Design review of the part built by this model. Coordinates are the model's own, in mm. Face numbers are marked on the shaded views. A direction names the side the tool comes from. Give positions to 0.01 mm unless a question says otherwise; leave off trailing zeros. Loops run counter-clockwise (first coordinate to the right, second up) from the corner with the lowest first, then second, coordinate; pieces in that order, holes last. Notation, with made-up numbers: (56, 19.5) -> (63, 19.5) arc R21 ccw to (63, 35.5) -> close; hole circle Ø2 at (59.25, -1). An arc over 180 degrees is marked (long way). Use a Markdown table: item, result. Add a question column.
1. Draft analysis for pull direction Y (two halves, no side actions). For the marked faces 1, 2 and 3, state which applies: pulls with the +Y half, pulls with the -Y half, needs draft (parallel to the pull), parting line crosses it, or undercut.
2. For pin 1 Ø1 at (y, z) = (17.5, 27.5) entering from +X; pin 2 Ø8 at (y, z) = (-16.5, 24) entering from +X; pin 3 Ø6 at (x, z) = (19, 27.5) entering from -Y, all flat-tipped, find the tip position at first contact; note any pin that passes through.
3. To check wall thickness, follow line 1 (Y direction, x = 0, z = 22.5); line 2 (Y direction, x = 0, z = 26.5); line 3 (X direction, y = -0.5, z = 15). State the ranges of each line that lie inside material, in increasing order.
4. Add section C-C (z = 12). Count the separate pieces of the cut face and the enclosed holes in it, and give its area (3 significant figures).
5. Add section D-D (x = 31.75). State the section outline as (y, z) points.
6. For the marked faces 4 and 5, list the 3-axis set-ups (+Z, -Z, +X, -X, +Y, -Y) from which the entire face can be reached by the end or side of a thin tool; tool diameter is ignored.
7. Add section A-A (x = 0). State the section outline as (y, z) points.
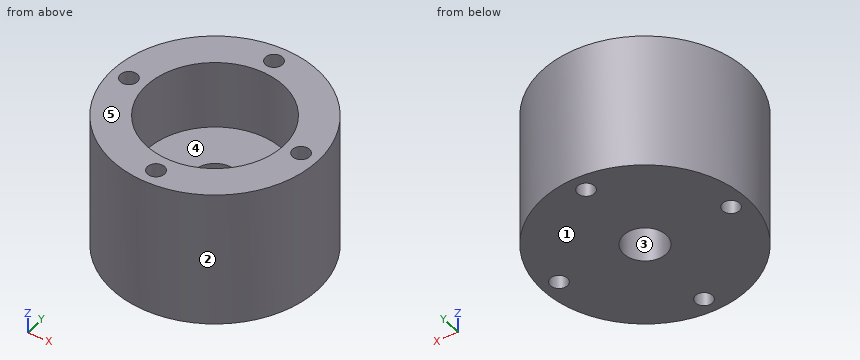
```python
from build123d import *

# Parameters (mm, degrees)
SKETCH1_R           = 38.1
BOSS_EXTRUDE1_DEPTH = 50.8
SKETCH2_R           = 7.9375
SKETCH2_R_2         = 3.1623
CUT_EXTRUDE1_DEPTH  = 50.8
SKETCH3_R           = 25.4
CUT_EXTRUDE2_DEPTH  = 25.4


with BuildPart() as part:
    # Sketch1 → Boss-Extrude1 (new body)
    with BuildSketch(Plane.XY):
        Circle(SKETCH1_R)
    extrude(amount=BOSS_EXTRUDE1_DEPTH)

    # Sketch2 → Cut-Extrude1 (cut)
    with BuildSketch(Plane.XY.offset(50.8)):
        Circle(SKETCH2_R)
        with Locations((0, 31.75)):
            Circle(SKETCH2_R_2)
        with Locations((0, -31.75)):
            Circle(SKETCH2_R_2)
        with Locations((31.75, 0)):
            Circle(SKETCH2_R_2)
        with Locations((-31.75, 0)):
            Circle(SKETCH2_R_2)
    extrude(amount=-CUT_EXTRUDE1_DEPTH, mode=Mode.SUBTRACT)

    # Sketch3 → Cut-Extrude2 (cut)
    with BuildSketch(Plane.XY.offset(50.8)):
        Circle(SKETCH3_R)
    extrude(amount=-CUT_EXTRUDE2_DEPTH, mode=Mode.SUBTRACT)


solid = part.part
```
Taken from the geometry:
| question | item | result |
|---|---|---|
| 1 | face 1 | needs draft |
| 1 | face 2 | parting line crosses it |
| 1 | face 3 | undercut |
| 2 | pin 1 | stops at x = 34.1 |
| 2 | pin 2 | stops at x = 35.99 |
| 2 | pin 3 | stops at y = -34.58 |
| 3 | line 1 | y = -38.1 to -34.91, -28.59 to -7.94, 7.94 to 28.59, 34.91 to 38.1 |
| 3 | line 2 | y = -38.1 to -34.91, -28.59 to -25.4, 25.4 to 28.59, 34.91 to 38.1 |
| 3 | line 3 | x = -38.1 to -34.87, -28.63 to -7.92, 7.92 to 28.63, 34.87 to 38.1 |
| 4 | separate pieces | 1 |
| 4 | enclosed holes | 5 |
| 4 | area | 4,240 mm^2 |
| 5 | outline | (-21.06, 0) -> (-3.16, 0) -> (-3.16, 50.8) -> (-21.06, 50.8) -> close; (3.16, 0) -> (21.06, 0) -> (21.06, 50.8) -> (3.16, 50.8) -> close |
| 6 | face 4 | +Z |
| 6 | face 5 | +Z, +X, -X, +Y, -Y |
| 7 | outline | (-38.1, 0) -> (-34.91, 0) -> (-34.91, 50.8) -> (-38.1, 50.8) -> close; (-28.59, 0) -> (-7.94, 0) -> (-7.94, 25.4) -> (-25.4, 25.4) -> (-25.4, 50.8) -> (-28.59, 50.8) -> close; (7.94, 0) -> (28.59, 0) -> (28.59, 50.8) -> (25.4, 50.8) -> (25.4, 25.4) -> (7.94, 25.4) -> close; (34.91, 0) -> (38.1, 0) -> (38.1, 50.8) -> (34.91, 50.8) -> close |
